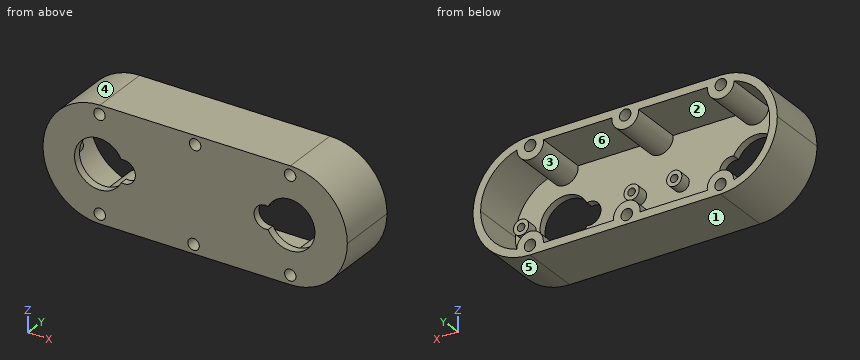
from build123d import *

# Parameters (mm, degrees)
SKETCH3_R            = 1.5
BOSS_EXTRUDE9_DEPTH  = 16
SHELL6_T             = -2
CUT_EXTRUDE3_DEPTH   = 16
SKETCH12_R           = 2
SKETCH12_R_2         = 1
BOSS_EXTRUDE16_DEPTH = 3


with BuildPart() as part:
    # Sketch3 → Boss-Extrude9 (new body)
    with BuildSketch(Plane(origin=(0, 0, 0), x_dir=(1, 0, 0), z_dir=(0, 1, 0))):
        with BuildLine():
            Line((-7.591309311, 15.762711864), (42.428690689, 15.762711864))
            ThreePointArc((42.428690689, 15.762711864), (53.028221339, 11.372242514), (57.418690689, 0.772711864))
            Line((57.418690689, 0.772711864), (57.418690689, 0.752711864))
            ThreePointArc((57.418690689, 0.752711864), (53.028221339, -9.846818786), (42.428690689, -14.237288136))
            Line((42.428690689, -14.237288136), (-7.591309311, -14.237288136))
            ThreePointArc((-7.591309311, -14.237288136), (-18.190839961, -9.846818786), (-22.581309311, 0.752711864))
            Line((-22.581309311, 0.752711864), (-22.581309311, 0.772711864))
            ThreePointArc((-22.581309311, 0.772711864), (-18.190839961, 11.372242514), (-7.591309311, 15.762711864))
        make_face()
        with Locations(Location((-7.655094993, 13.320472835, 0), (0, 0, 270))):
            Circle(SKETCH3_R, mode=Mode.SUBTRACT)
        with Locations(Location((-7.728737311, -11.852412523, 0), (0, 0, 270))):
            Circle(SKETCH3_R, mode=Mode.SUBTRACT)
        with Locations(Location((17.418690689, -11.898221857, 0), (0, 0, 270))):
            Circle(SKETCH3_R, mode=Mode.SUBTRACT)
        with Locations(Location((17.006406688, 13.388530255, 0), (0, 0, 270))):
            Circle(SKETCH3_R, mode=Mode.SUBTRACT)
        with Locations(Location((42.428690689, 13.342720921, 0), (0, 0, 270))):
            Circle(SKETCH3_R, mode=Mode.SUBTRACT)
        with Locations(Location((42.382881356, -11.852412523, 0), (0, 0, 270))):
            Circle(SKETCH3_R, mode=Mode.SUBTRACT)
    extrude(amount=BOSS_EXTRUDE9_DEPTH)

    # Shell6
    shell6_openings = [part.faces().sort_by_distance(p)[0] for p in [
        (17.420843578, 16, -0.763128508),
    ]]
    offset(amount=SHELL6_T, openings=shell6_openings)

    # Sketch6 → Cut-Extrude3 (cut)
    with BuildSketch(Plane(origin=(0, 2, 0), x_dir=(1, 0, 0), z_dir=(0, 1, 0))):
        with BuildLine():
            ThreePointArc((36.601110118, 3.632363117), (48.908802425, 0.713337584), (36.601110118, -2.205687948))
            ThreePointArc((36.601110118, -2.205687948), (32.908802425, 0.713337584), (36.601110118, 3.632363117))
        make_face()
        with BuildLine():
            ThreePointArc((-1.996728909, 3.621416563), (-14.304421217, 0.70239103), (-1.996728909, -2.216634502))
            ThreePointArc((-1.996728909, -2.216634502), (1.695578783, 0.70239103), (-1.996728909, 3.621416563))
        make_face()
    extrude(amount=-CUT_EXTRUDE3_DEPTH, mode=Mode.SUBTRACT)

    # Sketch12 → Boss-Extrude16 (add)
    with BuildSketch(Plane(origin=(0, 2, 0), x_dir=(1, 0, 0), z_dir=(0, 1, 0))):
        with Locations(Location((51.950259108, 0.701799296, 0), (0, 0, 270))):
            Circle(SKETCH12_R)
        with Locations(Location((51.950259108, 0.701799296, 0), (0, 0, 270))):
            Circle(SKETCH12_R_2, mode=Mode.SUBTRACT)
        with Locations(Location((-17.227337288, 0.701799296, 0), (0, 0, 270))):
            Circle(SKETCH12_R)
        with Locations(Location((-17.227337288, 0.701799296, 0), (0, 0, 270))):
            Circle(SKETCH12_R_2, mode=Mode.SUBTRACT)
        with Locations(Location((11.695578783, 0.70239103, 0), (0, 0, 270))):
            Circle(SKETCH12_R)
        with Locations(Location((11.695578783, 0.70239103, 0), (0, 0, 270))):
            Circle(SKETCH12_R_2, mode=Mode.SUBTRACT)
        with Locations(Location((22.908802425, 0.713337584, 0), (0, 0, 270))):
            Circle(SKETCH12_R)
        with Locations(Location((22.908802425, 0.713337584, 0), (0, 0, 270))):
            Circle(SKETCH12_R_2, mode=Mode.SUBTRACT)
    extrude(amount=BOSS_EXTRUDE16_DEPTH)


solid = part.part
The model under review builds one solid part; all positions refer to its coordinate system, in mm. Face numbers are marked on the shaded views. A direction names the side the tool comes from. Give positions to 0.01 mm unless a question says otherwise; leave off trailing zeros. Loops run counter-clockwise (first coordinate to the right, second up) from the corner with the lowest first, then second, coordinate; pieces in that order, holes last. Notation, with made-up numbers: (-19, 75.25) -> (27, 75.25) arc R25 ccw to (27, 110.25) -> close; hole circle Ø8 at (-3, 32). An arc over 180 degrees is marked (long way). Answer as a JSON object with one key per item and string values. Group by question number.
Q1. Insertion check: pin 1 (1.2 mm diameter, centred on x = 23, z = 0, fed in from +Y); pin 2 (1 mm diameter, centred on x = -17.5, z = -1, fed in from +Y); pin 3 (1.5 mm diameter, centred on x = -14, y = 2.5, fed in from -Z); pin 4 (3.5 mm diameter, centred on x = 35.91, z = -0.71, fed in from +Y). Each pin has a flat end and moves straight along its axis. Give the tip position at first contact, or say it passes through.
Q2. Take a section at B-B (x = 28.5). Write out the cut boundary in (y, z), plus the area to 3 significant figures.
Q3. Wall thickness on line 1 along Z through (x, y) = (-1, 14.25); line 2 along Z through (x, y) = (-7.5, 7.25); line 3 along X through (y, z) = (9, 12.5): over which ranges is each line inside the solid? List them lowest first.
Q4. Take a section at A-A (y = 10.5). State how many separate pieces and enclosed holes the cut face has, plus the area to 3 significant figures.
Q5. Draft analysis for pull direction X (two halves, no side actions). For the marked faces 1, 2, 3 and 4, state which applies: pulls with the +X half, pulls with the -X half, needs draft (parallel to the pull), parting line crosses it, or undercut.
Q6. Tool access review of the marked faces 5 and 6: name each direction out of +Z, -Z, +X, -X, +Y, -Y from which nothing blocks a thin tool from reaching the whole face with its end or side.
Answer below:
{
 "1": {"pin 1": "stops at y = 5", "pin 2": "stops at y = 2", "pin 3": "stops at z = -14.65", "pin 4": "passes through"},
 "2": {"outline": "(0, -15.76) -> (16, -15.76) -> (16, -13.76) -> (2, -13.76) -> (2, 12.24) -> (16, 12.24) -> (16, 14.24) -> (0, 14.24) -> close", "area": "116 mm2"},
 "3": {"line 1": "z = -15.76 to -13.76, 12.24 to 14.24", "line 2": "z = -15.76 to -14.81, -11.83 to -9.82, 8.36 to 10.37, 13.33 to 14.24", "line 3": "x = -14.6 to -9.08, -6.38 to 16.04, 18.79 to 41.03, 43.74 to 49.43"},
 "4": {"separate pieces": "1", "enclosed holes": "7", "area": "463 mm2"},
 "5": {"face 1": "needs draft", "face 2": "undercut", "face 3": "undercut", "face 4": "pulls with the -X half"},
 "6": {"face 5": "-Z, +X, +Y, -Y", "face 6": "+Y"}
}
